from build123d import *

# Parameters (mm, degrees)
F0_R     = 9.525
F0_R_2   = 12.7
F1_DEPTH = 19.05
F2_R     = 34.925
F2_R_2   = 12.7
F3_DEPTH = 19.05
F5_DEPTH = 12.7


with BuildPart() as f1:
    # F0 (on Top) → F1 (new body)
    with BuildSketch(Plane.XY):
        with BuildLine():
            Line((-37.419644, -16.497784), (0.680356, -38.494829))
            ThreePointArc((0.680356, -38.494829), (22.905356, -44.45), (45.130356, -38.494829))
            Line((45.130356, -38.494829), (83.230356, -16.497784))
            ThreePointArc((83.230356, -16.497784), (92.755356, 0), (83.230356, 16.497784))
            Line((83.230356, 16.497784), (45.130356, 38.494829))
            ThreePointArc((45.130356, 38.494829), (22.905356, 44.45), (0.680356, 38.494829))
            Line((0.680356, 38.494829), (-37.419644, 16.497784))
            ThreePointArc((-37.419644, 16.497784), (-46.944644, 0), (-37.419644, -16.497784))
        make_face()
        with Locations((-27.894644, 0)):
            Circle(F0_R, mode=Mode.SUBTRACT)
        with Locations((22.905356, 0)):
            Circle(F0_R_2, mode=Mode.SUBTRACT)
        with Locations((73.705356, 0)):
            Circle(F0_R, mode=Mode.SUBTRACT)
    extrude(amount=F1_DEPTH)

    # F2 (on face) → F3 (join)
    with BuildSketch(Plane.XY.offset(19.05)):
        with Locations((22.905356, 0)):
            Circle(F2_R)
        with Locations((22.905356, 0)):
            Circle(F2_R_2, mode=Mode.SUBTRACT)
    extrude(amount=F3_DEPTH)

    # F4 (on face) → F5 (join)
    with BuildSketch(Plane.XY.offset(38.1)):
        with BuildLine():
            Line((53.067856, 6.35), (57.248232, 6.35))
            ThreePointArc((57.248232, 6.35), (47.60106, 24.695704), (29.255356, 34.342876))
            Line((29.255356, 34.342876), (29.255356, 30.1625))
            Line((29.255356, 30.1625), (29.255356, 24.593444))
            ThreePointArc((29.255356, 24.593444), (40.865868, 17.960512), (47.4988, 6.35))
            Line((47.4988, 6.35), (53.067856, 6.35))
        make_face()
        with BuildLine():
            Line((29.255356, -24.593444), (29.255356, -30.1625))
            Line((29.255356, -30.1625), (29.255356, -34.342876))
            ThreePointArc((29.255356, -34.342876), (47.60106, -24.695704), (57.248232, -6.35))
            Line((57.248232, -6.35), (53.067856, -6.35))
            Line((53.067856, -6.35), (47.4988, -6.35))
            ThreePointArc((47.4988, -6.35), (40.865868, -17.960512), (29.255356, -24.593444))
        make_face()
        with BuildLine():
            Line((16.555356, -34.342876), (16.555356, -30.1625))
            Line((16.555356, -30.1625), (16.555356, -24.593444))
            ThreePointArc((16.555356, -24.593444), (4.944843, -17.960512), (-1.688089, -6.35))
            Line((-1.688089, -6.35), (-7.257144, -6.35))
            Line((-7.257144, -6.35), (-11.43752, -6.35))
            ThreePointArc((-11.43752, -6.35), (-1.790349, -24.695704), (16.555356, -34.342876))
        make_face()
        with BuildLine():
            Line((-11.43752, 6.35), (-7.257144, 6.35))
            Line((-7.257144, 6.35), (-1.688089, 6.35))
            ThreePointArc((-1.688089, 6.35), (4.944843, 17.960512), (16.555356, 24.593444))
            Line((16.555356, 24.593444), (16.555356, 30.1625))
            Line((16.555356, 30.1625), (16.555356, 34.342876))
            ThreePointArc((16.555356, 34.342876), (-1.790349, 24.695704), (-11.43752, 6.35))
        make_face()
    extrude(amount=F5_DEPTH)


solid = f1.part
Read the model definition and answer for the solid it produces. Units are mm, in the model's axes. A direction names the side the tool comes from. Round coordinates to 2 decimals unless told otherwise and drop trailing zeros. Write each loop counter-clockwise with the first axis right and the second up, starting at its lowest first coordinate (ties: lowest second). Pieces come first, ordered by that corner, then holes. Notation, with made-up numbers: (15, -21.5) - (20, -21.5) arc R27 cw to (20, 3.5) - close; hole circle Ø10 at (46, 77). An arc over 180 degrees is marked (long way). One line per question, with ' | ' between items. Start each with the question number.
1. Section D-D (x = 21.5) is taken. Determine the outline of the cut face in (y, z), and give its area (3 significant figures).
2. For a pull along X with two mould halves and no side action, classify faces 1 (the face through (52, -6.35, 44)), 2 (the face through (-18.1, 27.65, 9.39)), 3 (the face through (64.45, 27.34, 9.39)), 4 (the face through (4.811, 17.826, 44.361)) as +X half, -X half, draft (parallel to the pull), parting line (faces both ways), or undercut.
3. Find the intervals of material crossed by probe 1 along Z at (x, y) = (27, 21.5); probe 2 along Y at (x, z) = (69.5, 4) (3 decimals); probe 3 along X at (y, z) = (-4.5, 12.5), in increasing order. Write a range as [from, to].
4. Section B-B (z = 17.5) is taken. Determine the outline of the cut face in (x, y) (3 decimals), and give its area (3 significant figures).
5. Section C-C (y = 0) is taken. Determine the outline of the cut face in (x, z), and give its area (3 significant figures).
6. Section A-A (z = 39.5) is taken. Determine the outline of the cut face in (x, y) (3 decimals).
7. Each of these flat-tipped pins is pushed along its axis until it touches: pin 1 (22 mm diameter, centred on x = -27.89, y = 0, fed in from +Z); pin 2 (5 mm diameter, centred on x = -7.5, z = 43.5, fed in from -Y); pin 3 (3 mm diameter, centred on y = 30, z = 38, fed in from +X). Where does it stop, or does it pass through?
8. For faces 5 (the face through (-6, -6.35, 44)), 6 (the face through (7, 0, 38.1)), 7 (the face through (22.58, -44.45, 9.39)), 8 (the face through (16.555, -30, 44)), determine the directions among +Z, -Z, +X, -X, +Y, -Y from which every point of the face is accessible in a straight line to the end or side of a thin tool.
Filled in:
1) outline: (-44.43, 0) - (-12.62, 0) - (-12.62, 38.1) - (-34.9, 38.1) - (-34.9, 19.05) - (-44.43, 19.05) - close; (12.62, 0) - (44.43, 0) - (44.43, 19.05) - (34.9, 19.05) - (34.9, 38.1) - (12.62, 38.1) - close | area: 2,060 mm²
2) face 1: draft | face 2: -X half | face 3: +X half | face 4: undercut
3) probe 1: [0, 38.1] | probe 2: [-24.425, -8.546], [8.546, 24.425] | probe 3: [-46.41, -36.29], [-19.5, 11.03], [34.78, 65.31], [82.1, 92.22]
4) outline: (-37.42, -16.498) - (0.68, -38.495) arc R44.45 ccw to (45.13, -38.495) - (83.23, -16.498) arc R19.05 ccw to (83.23, 16.498) - (45.13, 38.495) arc R44.45 ccw to (0.68, 38.495) - (-37.42, 16.498) arc R19.05 ccw to start; hole circle Ø19.05 at (-27.895, 0); hole circle Ø25.4 at (22.905, 0); hole circle Ø19.05 at (73.705, 0) | area: 7,340 mm²
5) outline: (-46.94, 0) - (-37.42, 0) - (-37.42, 19.05) - (-46.94, 19.05) - close; (-18.37, 0) - (10.21, 0) - (10.21, 38.1) - (-12.02, 38.1) - (-12.02, 19.05) - (-18.37, 19.05) - close; (35.61, 0) - (64.18, 0) - (64.18, 19.05) - (57.83, 19.05) - (57.83, 38.1) - (35.61, 38.1) - close; (83.23, 0) - (92.76, 0) - (92.76, 19.05) - (83.23, 19.05) - close | area: 2,300 mm²
6) outline: (-11.438, -6.35) arc R34.925 ccw to (16.555, -34.343) - (16.555, -24.593) arc R25.4 cw to (-1.688, -6.35) - close; (-11.438, 6.35) - (-1.688, 6.35) arc R25.4 cw to (16.555, 24.593) - (16.555, 34.343) arc R34.925 ccw to start; (29.255, -34.343) arc R34.925 ccw to (57.248, -6.35) - (47.499, -6.35) arc R25.4 cw to (29.255, -24.593) - close; (29.255, 24.593) arc R25.4 cw to (47.499, 6.35) - (57.248, 6.35) arc R34.925 ccw to (29.255, 34.343) - close
7) pin 1: z = 19.05 | pin 2: y = -21 | pin 3: x = 43.09
8) face 5: +Z, +X, -X | face 6: +Z | face 7: +Z, -Z, -Y | face 8: +Z, +Y, -Y
